Build history of the part. All positions in model axes, mm. Face numbers are marked on the shaded views. A direction names the side the tool comes from. Round coordinates to 2 decimals unless told otherwise and drop trailing zeros. Order: outer loops, then holes, each group sorted by start corner. A loop starts at its lowest first (then second) coordinate and runs counter-clockwise, first axis right, second up. Notation, with made-up numbers: (-30, 48) - (-14, 48) arc R11 cw to (-14, 62) - close; hole circle Ø8 at (33, 10.25). An arc over 180 degrees is marked (long way). One line per question, with ' | ' between items. Start each with the question number.
Autodesk Inventor part; units mm, degrees
ref_plane "YZ Plane" through (0, 0, 0) normal (1, 0, 0) x (0, 1, 0)
ref_plane "XZ Plane" through (0, 0, 0) normal (0, 1, 0) x (-1, 0, 0)
ref_plane "XY Plane" through (0, 0, 0) normal (0, 0, 1) x (1, 0, 0)
sketch "Sketch1" plane through (0, 0, 0) normal (0, 0, 1) x (1, 0, 0)
  line L0 (-14, 0) -> (14, 0) construction
  line L1 (-14, -4) -> (14, -4)
  line L2 (14, 4) -> (-14, 4)
  arc A0 (-14, 4) -> (-14, -4) centre (-14, 0) ccw
  arc A1 (14, -4) -> (14, 4) centre (14, 0) ccw
  point P0 (0, 0)
  dimension "d0" = 8
  dimension "d1" = 28
extrude "Extrusion1" add sketch "Sketch1" along normal blind 7
sketch "Sketch2" plane through (-14, -4, 0) normal (0, -1, 0) x (1, 0, 0)
  line L0 (7.5, 0) -> (20.5, 0) construction
  line L1 (7.5, -4) -> (20.5, -4)
  line L2 (20.5, 4) -> (7.5, 4)
  arc A0 (7.5, 4) -> (7.5, -4) centre (7.5, 0) ccw
  arc A1 (20.5, -4) -> (20.5, 4) centre (20.5, 0) ccw
  point P0 (14, 0)
  dimension "d4" = 4
  dimension "d5" = 13
extrude "Extrusion2" cut sketch "Sketch2" against normal through all
fillet "Fillet1" radius 1.5 6 edges at (0, -4, 4) (9.3284, -4, 2.8284) (-9.3284, -4, 2.8284) (0, 4, 4) (9.3284, 4, 2.8284) (-9.3284, 4, 2.8284)
fillet "Fillet2" radius 1 4 edges at (18, 0, 7) (0, 4, 7) (-18, 0, 7) (0, -4, 7)
sketch "Sketch3" plane through (0, 0, 7) normal (0, 0, 1) x (1, 0, 0)
  arc A0 (14, -4) -> (14, 4) centre (14, 0) ccw
  arc A1 (-14, 4) -> (-14, -4) centre (-14, 0) ccw
  point P0 (0, 0)
hole "Hole1" at (14, 0, 7) at (-14, 0, 7) direction (0, 0, -1) diameter 1.9 end through all counterbore diameter 4 counterbore depth 4
properties part number "cable clip"
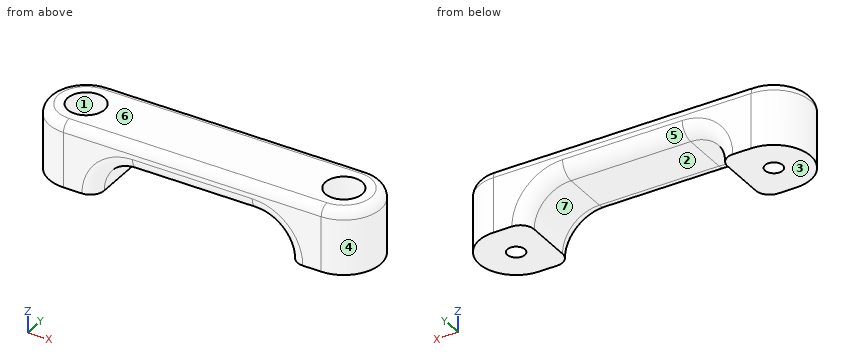
Item 1: Slice it at B-B (z = 1.75). Count the separate pieces of the cut face and the enclosed holes in it, plus the area to 3 significant figures.
Item 2: Pull direction X, two halves, no side cores. Call the marked faces 4, 5, 6 and 7: released by +X, released by -X, zero draft, split by the parting line, or undercut.
Item 3: 3-axis set-ups, long thin cutter, end or side, ignore diameter. For the marked faces 1, 2 and 3: which of +Z, -Z, +X, -X, +Y, -Y reach the whole face in a straight line?
Item 4: Slice it at A-A (y = 0). Write the cut outline in (x, z).
Item 5: Wall check: line 1 along X through (y, z) = (0, 4.25); line 2 along Y through (x, z) = (-14, 1.25); line 3 along X through (y, z) = (0, 1.65). Give the ranges that are in metal, low to high. Write a range as [from, to].
Item 6: Pin check, flat tips, straight feed: pin 1 (1.2 mm diameter, centred on x = -14, y = 1, fed in from +Z); pin 2 (1 mm diameter, centred on x = -0.5, z = 4.5, fed in from +Y). Stop position of each tip, or through.
A:
1) separate pieces: 2 | enclosed holes: 2 | area: 105 mm^2
2) face 4: released by +X | face 5: undercut | face 6: zero draft | face 7: undercut
3) face 1: +Z | face 2: -Z, +Y, -Y | face 3: -Z, +X, -X, +Y, -Y
4) outline: (-18, 0) - (-14.95, 0) - (-14.95, 3) - (-16, 3) - (-16, 7) - (-17, 7) arc R1 ccw to (-18, 6) - close; (-13.05, 0) - (-10.5, 0) arc R4 cw to (-6.5, 4) - (6.5, 4) arc R4 cw to (10.5, 0) - (13.05, 0) - (13.05, 3) - (12, 3) - (12, 7) - (-12, 7) - (-12, 3) - (-13.05, 3) - close; (14.95, 0) - (18, 0) - (18, 6) arc R1 ccw to (17, 7) - (16, 7) - (16, 3) - (14.95, 3) - close
5) line 1: [-18, -16], [-12, 12], [16, 18] | line 2: [-4, -0.95], [0.95, 4] | line 3: [-18, -14.95], [-13.05, -10.14], [10.14, 13.05], [14.95, 18]
6) pin 1: z = 3 | pin 2: y = 3.91
